Design review of the part built by this model. Coordinates are the model's own, in mm. Coordinates: 2 decimals unless noted, no trailing zeros. Write each loop counter-clockwise with the first axis right and the second up, starting at its lowest first coordinate (ties: lowest second). Pieces come first, ordered by that corner, then holes.
Q1. Take a section at A-A, the plane x = 0. Write out the cut boundary in (y, z).
Q2. Take a section at C-C, the plane z = 31. Write out the cut boundary in (x, y).
Q3. For pin 1 Ø12 at (x, z) = (-5, 33.5) entering from +Y; pin 2 Ø6 at (x, z) = (5, 4.5) entering from +Y; pin 3 Ø6 at (y, z) = (6, 21.5) entering from +X; pin 4 Ø1 at (y, z) = (6, 17) entering from -X, all flat-tipped, find the tip position at first contact; note any pin that passes through.
Q4. For L1, parallel to Y at x = 0, z = 23; L2, parallel to Z at x = -3, y = 0.75; L3, parallel to Y at x = -5.5, z = 23, list the stretches that pass through material, from the lowest coordinate up.
Q5. The part is to be moulded in two halves that separate along X. For faces 1 (the cylindrical face through (-5.158, -3.955, 22.502)), 2 (the flat face through (0, 0, 0)), 3 (the cylindrical face through (10, 3.2, 20)), say which applies: released by +X, released by -X, zero draft, split by the parting line, or undercut.
from build123d import *

# Parameters (mm, degrees)
SKETCH1_R           = 10.5
BOSS_EXTRUDE1_DEPTH = 40.5
SHELL1_T            = -4
FILLET1_R           = 3.5
FILLET2_R           = 3.5
FILLET3_R           = 1


with BuildPart() as part:
    # Sketch1 → Boss-Extrude1 (new body)
    with BuildSketch(Plane.XY):
        Circle(SKETCH1_R)
    extrude(amount=BOSS_EXTRUDE1_DEPTH)

    # Shell1
    shell1_openings = [part.faces().sort_by_distance(p)[0] for p in [
        (0, 0, 40.5),
    ]]
    offset(amount=SHELL1_T, openings=shell1_openings, kind=Kind.INTERSECTION)

    # Fillet1
    fillet1_edges = [part.edges().sort_by_distance(p)[0] for p in [
        (-10.5, 0, 40.5),
    ]]
    fillet(fillet1_edges, radius=FILLET1_R)

    # Fillet2
    fillet2_edges = [part.edges().sort_by_distance(p)[0] for p in [
        (-10.5, 0, 0),
    ]]
    fillet(fillet2_edges, radius=FILLET2_R)

    # Fillet3
    fillet3_edges = [part.edges().sort_by_distance(p)[0] for p in [
        (-6.5, 0, 4),
    ]]
    fillet(fillet3_edges, radius=FILLET3_R)


solid = part.part
Responses:
1. outline: (-10.5, 3.5) arc R3.5 ccw to (-7, 0) - (7, 0) arc R3.5 ccw to (10.5, 3.5) - (10.5, 37) arc R3.5 ccw to (7, 40.5) - (6.5, 40.5) - (6.5, 5) arc R1 cw to (5.5, 4) - (-5.5, 4) arc R1 cw to (-6.5, 5) - (-6.5, 40.5) - (-7, 40.5) arc R3.5 ccw to (-10.5, 37) - close
2. outline: circle Ø21 at (0, 0); hole circle Ø13 at (0, 0)
3. pin 1: stops at y = 10.5
3. pin 2: stops at y = 10.31
3. pin 3: stops at x = 10.06
3. pin 4: stops at x = -8.94
4. L1: y = -10.5 to -6.5, 6.5 to 10.5
4. L2: z = 0 to 4
4. L3: y = -8.94 to -3.46, 3.46 to 8.94
5. face 1: undercut
5. face 2: zero draft
5. face 3: split by the parting line
